Geometry: final body of the model. Coordinates: model frame, mm. A direction names the side the tool comes from. Coordinates: 2 decimals unless noted, no trailing zeros. Loops run counter-clockwise (first coordinate to the right, second up) from the corner with the lowest first, then second, coordinate; pieces in that order, holes last. Notation, with made-up numbers: (-2.5, 28) - (26.5, 28) arc R25 ccw to (26.5, 65) - close; hole circle Ø4 at (86, -26). An arc over 180 degrees is marked (long way). Return JSON: item names as keys, results as strings.
from build123d import *

# Parameters (mm, degrees)
F0_R     = 6.35
F1_DEPTH = 31.75
F3_DEPTH = 127


with BuildPart() as f1:
    # F0 (on Front) → F1 (new body)
    with BuildSketch(Plane.XZ):
        with BuildLine():
            Line((-61.976, 16.002), (-61.976, 0))
            Line((-61.976, 0), (61.976, 0))
            Line((61.976, 0), (61.976, 16.002))
            Line((61.976, 16.002), (30.226, 16.002))
            Line((30.226, 16.002), (26.391128, 34.989695))
            ThreePointArc((26.391128, 34.989695), (0, 56.58358), (-26.391128, 34.989695))
            Line((-26.391128, 34.989695), (-30.226, 16.002))
            Line((-30.226, 16.002), (-61.976, 16.002))
        make_face()
        with Locations((0, 30.226)):
            Circle(F0_R, mode=Mode.SUBTRACT)
    extrude(amount=F1_DEPTH)

    # F2 (on face) → F3 (cut)
    with BuildSketch(Plane(origin=(0, 0, 0), x_dir=(1, 0, 0), z_dir=(0, 0, -1))):
        with BuildLine():
            Line((-38.1, 21.463), (-50.038, 21.463))
            ThreePointArc((-50.038, 21.463), (-55.626, 15.875), (-50.038, 10.287))
            Line((-50.038, 10.287), (-38.1, 10.287))
            ThreePointArc((-38.1, 10.287), (-32.512, 15.875), (-38.1, 21.463))
        make_face()
        with BuildLine():
            Line((50.038, 21.463), (38.1, 21.463))
            ThreePointArc((38.1, 21.463), (32.512, 15.875), (38.1, 10.287))
            Line((38.1, 10.287), (50.038, 10.287))
            ThreePointArc((50.038, 10.287), (55.626, 15.875), (50.038, 21.463))
        make_face()
    extrude(amount=-F3_DEPTH, mode=Mode.SUBTRACT)


solid = f1.part
Item 1: Ray query, probe 1 along Z at (x, y) = (-0.5, -25); probe 2 along Z at (x, y) = (-54, -22); probe 3 along X at (y, z) = (-20, 15.5). Return the intervals inside material, ascending. Write a range as from..to.
Worked out:
{"probe 1": "0..23.9, 36.56..56.58", "probe 2": "0..16", "probe 3": "-61.98..-53.81, -34.33..34.33, 53.81..61.98"}
Item 2: Section query C-C, the plane y = -15.5. Return loops of the section in (x, z), and give its area (3 significant figures).
Worked out:
{"outline": "(-61.98, 0) - (-55.61, 0) - (-55.61, 16) - (-61.98, 16) - close; (-32.52, 0) - (32.52, 0) - (32.52, 16) - (30.23, 16) - (26.39, 34.99) arc R26.92 ccw to (-26.39, 34.99) - (-30.23, 16) - (-32.52, 16) - close; (55.61, 0) - (61.98, 0) - (61.98, 16) - (55.61, 16) - close; hole circle Ø12.7 at (0, 30.23)", "area": "3,050 mm^2"}
Item 3: Section query B-B, the plane y = -3. Return loops of the section in (x, z).
Worked out:
{"outline": "(-61.98, 0) - (61.98, 0) - (61.98, 16) - (30.23, 16) - (26.39, 34.99) arc R26.92 ccw to (-26.39, 34.99) - (-30.23, 16) - (-61.98, 16) - close; hole circle Ø12.7 at (0, 30.23)"}
Item 4: Reachability of faces 1 (the face through (0.52, -15.65, 56.58)), 2 (the face through (-32.513, -15.752, 7.889)), 3 (the face through (46, -23, 16.002)), 4 (the face through (-1, -31.75, 22)), 5 (the face through (-46, -23, 16.002)) from +Z, -Z, +X, -X, +Y, -Y: full face, straight path, thin tool, end or side. Return the list, or none.
Worked out:
{"face 1": "+Z, +Y, -Y", "face 2": "+Z, -Z", "face 3": "+Z, +X, +Y, -Y", "face 4": "+Z, -Z, +X, -X, -Y", "face 5": "+Z, -X, +Y, -Y"}
Item 5: First-contact query: pin 1 Ø5 at (x, z) = (2.5, 29.5) entering from +Y; pin 2 Ø20.5 at (x, z) = (0, 30.226) entering from +Y; pin 3 Ø2 at (y, z) = (-6.5, 47.5) entering from +X; pin 4 Ø16 at (x, y) = (50.5, -17.5) entering from +Z. Flat tips, straight axial feed; report the tip coordinate or a pass-through.
Worked out:
{"pin 1": "through", "pin 2": "y = 0", "pin 3": "x = 21.01", "pin 4": "z = 16"}
Item 6: Section query D-D, the plane z = 7. Return loops of the section in (x, y) (3 decimals), and give its area (3 significant figures).
Worked out:
{"outline": "(-61.976, -31.75) - (61.976, -31.75) - (61.976, 0) - (-61.976, 0) - close; hole (-50.038, -21.463) - (-38.1, -21.463) arc R5.588 ccw to (-38.1, -10.287) - (-50.038, -10.287) arc R5.588 ccw to start; hole (38.1, -21.463) - (50.038, -21.463) arc R5.588 ccw to (50.038, -10.287) - (38.1, -10.287) arc R5.588 ccw to start", "area": "3,470 mm^2"}
Item 7: Mould query, pull axis X, two halves, no side actions, for faces 6 (the face through (-28.28, -15.65, 25.63)), 7 (the face through (-44, -10.287, 8)), 8 (the face through (-1, 0, 22)). Classes: +X half, -X half, draft (parallel to the pull), parting line (faces both ways), or undercut.
Worked out:
{"face 6": "-X half", "face 7": "undercut", "face 8": "draft"}
Item 8: Section query A-A, the plane x = -40. Return loops of the section in (y, z).
Worked out:
{"outline": "(-31.75, 0) - (-21.46, 0) - (-21.46, 16) - (-31.75, 16) - close; (-10.29, 0) - (0, 0) - (0, 16) - (-10.29, 16) - close"}
